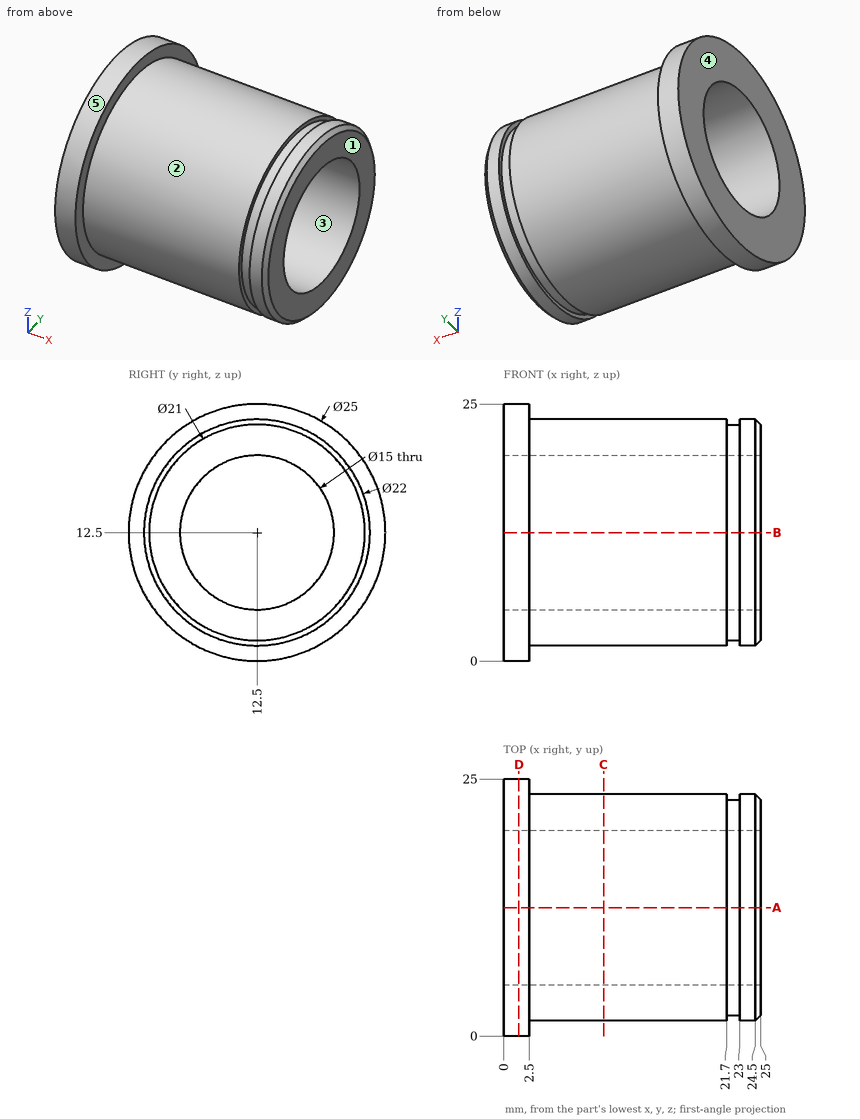
Part print with two shaded views. Sizes in mm from the minimum x, y, z corner. A direction names the side the tool comes from. Round coordinates to 2 decimals unless told otherwise and drop trailing zeros. Loops run counter-clockwise (first coordinate to the right, second up) from the corner with the lowest first, then second, coordinate; pieces in that order, holes last. Notation, with made-up numbers: (-10.5, 8.25) - (22.5, 8.25) arc R37 cw to (22.5, 44.25) - close; hole circle Ø10 at (-32.75, 33.5). An arc over 180 degrees is marked (long way). Answer as a JSON object with one key per item and string values.
Item 1: Pin check, flat tips, straight feed: pin 1 (12 mm diameter, centred on x = 8, z = 5, fed in from -Y); pin 2 (1.5 mm diameter, centred on x = 19, y = 13.5, fed in from -Z); pin 3 (2 mm diameter, centred on x = 20, z = 16, fed in from -Y). Stop position of each tip, or through.
Output:
{"pin 1": "y = 1.09", "pin 2": "z = 1.5", "pin 3": "y = 1.79"}
Item 2: Tool access for the marked faces 1 and 2: list every direction of +Z, -Z, +X, -X, +Y, -Y with a clear straight run to the whole face (end or side of a thin tool).
Output:
{"face 1": "+Z, -Z, +X, +Y, -Y", "face 2": "+X"}
Item 3: Band-saw the part on A-A on y = 12.5. List the corners of the cut face in (x, z).
Output:
{"outline": "(0, 0) - (2.5, 0) - (2.5, 1.5) - (21.7, 1.5) - (21.7, 2) - (23, 2) - (23, 1.5) - (24.5, 1.5) - (25, 2) - (25, 5) - (0, 5) - close; (0, 20) - (25, 20) - (25, 23) - (24.5, 23.5) - (23, 23.5) - (23, 23) - (21.7, 23) - (21.7, 23.5) - (2.5, 23.5) - (2.5, 25) - (0, 25) - close"}
Item 4: Band-saw the part on C-C on x = 9.75. List the corners of the cut face in (y, z), plus the area to 3 significant figures.
Output:
{"outline": "circle Ø22 at (12.5, 12.5); hole circle Ø15 at (12.5, 12.5)", "area": "203 mm2"}
Item 5: Pull direction Y, two halves, no side cores. Call the marked faces 3, 4 and 5: pulls with the +Y half, pulls with the -Y half, needs draft (parallel to the pull), parting line crosses it, or undercut.
Output:
{"face 3": "undercut", "face 4": "needs draft", "face 5": "parting line crosses it"}
Item 6: Wall check: L1, parallel to Z at x = 16.25, y = 12.5; L2, parallel to Z at x = 23.25, y = 6.25; L3, parallel to Y at x = 4.75, z = 7.5. Give the ranges that are in metal, low to high.
Output:
{"L1": "1.5 to 5, 20 to 23.5", "L2": "3.45 to 8.35, 16.65 to 21.55", "L3": "2.7 to 6.91, 18.09 to 22.3"}
Item 7: Band-saw the part on D-D on x = 1.5. List the corners of the cut face in (y, z), plus the area to 3 significant figures.
Output:
{"outline": "circle Ø25 at (12.5, 12.5); hole circle Ø15 at (12.5, 12.5)", "area": "314 mm2"}
